Source: CAD feature listing. Evaluate the final solid. Frame: model axes, mm. A direction names the side the tool comes from. Coordinates: 2 decimals unless noted, no trailing zeros. Order: outer loops, then holes, each group sorted by start corner. A loop starts at its lowest first (then second) coordinate and runs counter-clockwise, first axis right, second up. Notation, with made-up numbers: (-34.75, -40) - (24.25, -40) arc R10 cw to (24.25, -36) - close; hole circle Ø3 at (-18, 2). An arc over 180 degrees is marked (long way). One line per question, with ' | ' between items.
from build123d import *

# Parameters (mm, degrees)
SKETCH1_R           = 18.5
BOSS_EXTRUDE1_DEPTH = 19.05
SKETCH2_R           = 16.5
BOSS_EXTRUDE2_DEPTH = 22.95
SKETCH3_R           = 4.5
BOSS_EXTRUDE3_DEPTH = 3
SKETCH4_R           = 1
BOSS_EXTRUDE4_DEPTH = 13.5
SKETCH5_R           = 6
BOSS_EXTRUDE5_DEPTH = 4.6
SKETCH7_R           = 3
BOSS_EXTRUDE6_DEPTH = 6
BOSS_EXTRUDE7_DEPTH = 12


with BuildPart() as part:
    # Sketch1 → Boss-Extrude1 (new body)
    with BuildSketch(Plane(origin=(0, 0, 0), x_dir=(0, 0, -1), z_dir=(1, 0, 0))):
        with Locations(Location((0, 0, 0), (0, 0, 180))):
            Circle(SKETCH1_R)
    extrude(amount=BOSS_EXTRUDE1_DEPTH)

    # Sketch2 → Boss-Extrude2 (add)
    with BuildSketch(Plane(origin=(19.05, 0, 0), x_dir=(0, 0, -1), z_dir=(1, 0, 0))):
        Circle(SKETCH2_R)
    extrude(amount=BOSS_EXTRUDE2_DEPTH)

    # Sketch3 → Boss-Extrude3 (add)
    with BuildSketch(Plane(origin=(42, 0, 0), x_dir=(0, 0, -1), z_dir=(1, 0, 0))):
        Circle(SKETCH3_R)
    extrude(amount=BOSS_EXTRUDE3_DEPTH)

    # Sketch4 → Boss-Extrude4 (add)
    with BuildSketch(Plane(origin=(45, 0, 0), x_dir=(0, 0, -1), z_dir=(1, 0, 0))):
        Circle(SKETCH4_R)
    extrude(amount=BOSS_EXTRUDE4_DEPTH)

    # Sketch5 → Boss-Extrude5 (add)
    with BuildSketch(Plane.ZY):
        with Locations(Location((0, -7, 0), (0, 0, 180))):
            Circle(SKETCH5_R)
    extrude(amount=BOSS_EXTRUDE5_DEPTH)

    # Sketch7 → Boss-Extrude6 (add)
    with BuildSketch(Plane.ZY.offset(4.6)):
        with Locations((0, -7)):
            Circle(SKETCH7_R)
    extrude(amount=BOSS_EXTRUDE6_DEPTH)

    # Sketch8 → Boss-Extrude7 (add)
    with BuildSketch(Plane.ZY.offset(10.6)):
        with BuildLine():
            Line((-1.658312395, -4.5), (1.658312395, -4.5))
            ThreePointArc((1.658312395, -4.5), (0, -10), (-1.658312395, -4.5))
        make_face()
    extrude(amount=BOSS_EXTRUDE7_DEPTH)


solid = part.part
(1) Cut plane D-D (z = 10). Return the cut outline in (x, y).
Taken from the geometry:
outline: (0, -15.56) - (19.05, -15.56) - (19.05, -13.12) - (42, -13.12) - (42, 13.12) - (19.05, 13.12) - (19.05, 15.56) - (0, 15.56) - close
(2) Cut plane C-C (x = -12.5). Return the cut outline in (y, z).
Taken from the geometry:
outline: (-4.5, -1.66) - (-4.5, 1.66) arc R3 ccw (long way) to start
(3) Cut plane A-A (y = 0). Return the cut outline in (x, z), and give its area (3 significant figures).
Taken from the geometry:
outline: (0, -18.5) - (19.05, -18.5) - (19.05, -16.5) - (42, -16.5) - (42, -4.5) - (45, -4.5) - (45, -1) - (58.5, -1) - (58.5, 1) - (45, 1) - (45, 4.5) - (42, 4.5) - (42, 16.5) - (19.05, 16.5) - (19.05, 18.5) - (0, 18.5) - close | area: 1,520 mm²
(4) Material intervals for L1, parallel to X at y = 1.5, z = -10.5; L2, parallel to X at y = 12, z = 14; L3, parallel to Y at x = 3, z = 0, sorted ascending. Write a range as from..to.
Taken from the geometry:
L1: x = 0..42 | L2: x = 0..19.05 | L3: y = -18.5..18.5
(5) Cut plane B-B (z = 0). Return the cut outline in (x, y), and give its area (3 significant figures).
Taken from the geometry:
outline: (-22.6, -10) - (-4.6, -10) - (-4.6, -13) - (0, -13) - (0, -18.5) - (19.05, -18.5) - (19.05, -16.5) - (42, -16.5) - (42, -4.5) - (45, -4.5) - (45, -1) - (58.5, -1) - (58.5, 1) - (45, 1) - (45, 4.5) - (42, 4.5) - (42, 16.5) - (19.05, 16.5) - (19.05, 18.5) - (0, 18.5) - (0, -1) - (-4.6, -1) - (-4.6, -4) - (-10.6, -4) - (-10.6, -4.5) - (-22.6, -4.5) - close | area: 1,670 mm²
(6) Set-up query: faces 1 (the cylindrical face through (52, -1, 0)), 2 (the flat face through (-4.6, -10, -1)), 3 (the flat face through (-17, -4.5, 0)). Return all of +Z, -Z, +X, -X, +Y, -Y with unobstructed straight access to the full face (end or side cutting, diameter ignored); none if empty.
Taken from the geometry:
face 1: +X | face 2: -X | face 3: +Z, -Z, -X, +Y
(7) Pin query (flat end, axial travel): P1, Ø6, axis at x = 17.5, y = 10, coming from the +Z side; P2, Ø12, axis at y = -3, z = -11, coming from the -X side; P3, Ø2, axis at x = 15, y = 1.5, coming from the +Z side. Return the tip coordinate at first contact, or that it passes through.
Taken from the geometry:
P1: stops at z = 17.12 | P2: stops at x = -4.6 | P3: stops at z = 18.49
